from build123d import *

# Parameters (mm, degrees)
F0_R     = 31.75
F1_DEPTH = 25.4
F2_DEPTH = 12.7
F4_DEPTH = 25.4


with BuildPart() as f1:
    # F0 (on Front) → F1 (new body)
    with BuildSketch(Plane.XZ):
        with BuildLine():
            ThreePointArc((40.001993, -10.986297), (41.111251, -5.542851), (41.483227, 0))
            ThreePointArc((41.483227, 0), (-5.542851, 41.111251), (-40.001993, -10.986297))
            ThreePointArc((-40.001993, -10.986297), (0, -41.483227), (40.001993, -10.986297))
        make_face()
        Circle(F0_R, mode=Mode.SUBTRACT)
    extrude(amount=F1_DEPTH)

    # F0 (on Front) → F2 (join)
    with BuildSketch(Plane.XZ):
        with BuildLine():
            ThreePointArc((40.001993, -10.986297), (41.111251, -5.542851), (41.483227, 0))
            ThreePointArc((41.483227, 0), (-5.542851, 41.111251), (-40.001993, -10.986297))
            ThreePointArc((-40.001993, -10.986297), (0, -41.483227), (40.001993, -10.986297))
        make_face()
        Circle(F0_R, mode=Mode.SUBTRACT)
        with BuildLine():
            ThreePointArc((40.001993, -10.986297), (0, -41.483227), (-40.001993, -10.986297))
            Line((-40.001993, -10.986297), (0, -156.636773))
            Line((0, -156.636773), (40.001993, -10.986297))
        make_face()
    extrude(amount=F2_DEPTH)

    # F3 (on face) → F4 (join)
    with BuildSketch(Plane(origin=(0, 0, 0), x_dir=(-1, 0, 0), z_dir=(0, 1, 0))):
        Polygon((5.272433, -37.112545), (-5.63112, -37.112545), (0, -156.636773), align=None)
    extrude(amount=-F4_DEPTH)


solid = f1.part
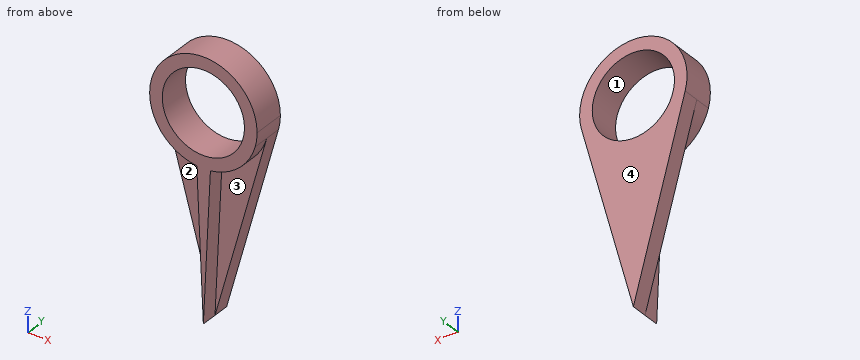
The listing builds one solid part. Answer for the finished solid, in the listing's coordinates (mm). Face numbers are marked on the shaded views. A direction names the side the tool comes from. Give positions to 0.01 mm unless a question says otherwise; leave off trailing zeros. Write each loop counter-clockwise with the first axis right and the second up, starting at its lowest first coordinate (ties: lowest second). Pieces come first, ordered by that corner, then holes.
1) Section D-D (z = -37) is taken. Write down the section's boundary in (x, y).
2) Given P1, Ø8, axis at x = -17.5, z = -76.5, coming from the -Y side; P2, Ø1.5, axis at x = 6, y = -5.5, coming from the +Z side; P3, Ø2, axis at y = -22.5, z = 17, coming from the -X side, each flat-ended and moving along its own axis, determine where each tip first touches the part or whether it passes through.
3) For a pull along X with two mould halves and no side action, classify the marked faces 1 and 2 as pulls with the +X half, pulls with the -X half, needs draft (parallel to the pull), parting line crosses it, or undercut.
4) Section A-A (z = 27) is taken. Write down the section's boundary in (x, y).
5) Find the intervals of material crossed by L1, parallel to Y at x = -3, z = -143; L2, parallel to Z at x = 10.5, y = -24; L3, parallel to X at y = -18.75, z = -28.5, in increasing order.
6) A tool of negligible diameter and unlimited length cuts with its end or side. For the marked faces 3 and 4, from which of +Z, -Z, +X, -X, +Y, -Y can it reach the whole face along a straight path? Write none if from no direction.
7) Section B-B (x = -19.5) is taken. Write down the section's boundary in (y, z), and give its area (3 significant figures).
8) Section C-C (y = -9) is taken. Write down the section's boundary in (x, z), and give its area (3 significant figures).
Response:
1. outline: (-32.86, -12.7) - (-18.76, -12.7) - (-18.76, -25.4) - (18.76, -25.4) - (18.76, -12.7) - (32.86, -12.7) - (32.86, 0) - (-32.86, 0) - close
2. P1: stops at y = -12.7
2. P2: stops at z = 41.15
2. P3: stops at x = -38.27
3. face 1: undercut
3. face 2: needs draft
4. outline: (-31.49, -25.4) - (-16.71, -25.4) - (-16.71, 0) - (-31.49, 0) - close; (16.71, -25.4) - (31.49, -25.4) - (31.49, 0) - (16.71, 0) - close
5. L1: y = -12.7 to 0
5. L2: z = -40.13 to -29.96, 29.96 to 40.13
5. L3: x = -30.14 to -13.99, 13.99 to 30.14
6. face 3: -Z, +X, -Y
6. face 4: +Z, -Z, +X, -X, +Y
7. outline: (-25.4, -36.61) - (-12.7, -36.61) - (-12.7, -85.64) - (0, -85.64) - (0, -25.06) - (-25.4, -25.06) - close; (-25.4, 25.06) - (0, 25.06) - (0, 36.61) - (-25.4, 36.61) - close
7. area: 1,210 mm2
8. outline: (-40, -10.99) - (0, -156.64) - (40, -10.99) arc R41.48 ccw to (41.48, 0) arc R41.48 ccw (long way) to start; hole circle Ø63.5 at (0, 0)
8. area: 6,260 mm2
